from build123d import *

# Parameters (mm, degrees)
SKETCH1_W           = 95.25
SKETCH1_H           = 12.8
BOSS_EXTRUDE1_DEPTH = 161.88
SKETCH1_3_R         = 3.1
CUT_EXTRUDE1_DEPTH  = 20.2
SKETCH1_4_R         = 2.395
CUT_EXTRUDE2_DEPTH  = 21.5
CUT_EXTRUDE3_REACH  = 14.8
SKETCH2_R           = 9.525
CUT_EXTRUDE4_REACH  = 14.8
SKETCH3_R           = 3.265
SKETCH3_R_2         = 1.96
SKETCH3_R_3         = 2.56
SKETCH4_R           = 9.525
SKETCH4_R_2         = 5.09
CUT_EXTRUDE5_DEPTH  = 3.32
SKETCH5_R           = 5.31
CUT_EXTRUDE6_DEPTH  = 6.65
SKETCH6_R           = 1.965
CUT_EXTRUDE7_DEPTH  = 17.25
SKETCH7_R           = 1.97
CUT_EXTRUDE8_DEPTH  = 15.87
SKETCH9_R           = 9.5
CUT_EXTRUDE9_DEPTH  = 13.8000001


with BuildPart() as part:
    # Sketch1 → Boss-Extrude1 (new body)
    with BuildSketch(Plane.XY):
        with Locations((-282.25, -616.5)):
            Rectangle(SKETCH1_W, SKETCH1_H)
    extrude(amount=BOSS_EXTRUDE1_DEPTH)

    # Sketch1_3 → Cut-Extrude1 (cut)
    with BuildSketch(Plane.XY):
        with Locations((-307.5, -616.5)):
            Circle(SKETCH1_3_R)
        with Locations((-257, -616.5)):
            Circle(SKETCH1_3_R)
    extrude(amount=CUT_EXTRUDE1_DEPTH, mode=Mode.SUBTRACT)

    # Sketch1_4 → Cut-Extrude2 (cut)
    with BuildSketch(Plane.XY):
        with Locations((-244.2, -616.5)):
            Circle(SKETCH1_4_R)
        with Locations((-320.5, -616.5)):
            Circle(SKETCH1_4_R)
    extrude(amount=CUT_EXTRUDE2_DEPTH, mode=Mode.SUBTRACT)

    # Sketch2 → Cut-Extrude3 (cut, up to next)
    with BuildSketch(Plane(origin=(0, -610.1, 0), x_dir=(1, 0, 0), z_dir=(0, 1, 0)), mode=Mode.PRIVATE) as cut_extrude3_sk1:
        with Locations((-275.57, -124.135)):
            Circle(SKETCH2_R)
    cut_extrude3_tool1 = extrude(cut_extrude3_sk1.sketch, amount=-CUT_EXTRUDE3_REACH, mode=Mode.PRIVATE) & part.part
    add(cut_extrude3_tool1.solids().sort_by_distance((-275.57, -610.1, 124.135))[0], mode=Mode.SUBTRACT)
    # Sketch2 → Cut-Extrude3 (cut, up to next)
    with BuildSketch(Plane(origin=(0, -610.1, 0), x_dir=(1, 0, 0), z_dir=(0, 1, 0)), mode=Mode.PRIVATE) as cut_extrude3_sk2:
        with Locations((-275.57, -86.105)):
            Circle(SKETCH2_R)
    cut_extrude3_tool2 = extrude(cut_extrude3_sk2.sketch, amount=-CUT_EXTRUDE3_REACH, mode=Mode.PRIVATE) & part.part
    add(cut_extrude3_tool2.solids().sort_by_distance((-275.57, -610.1, 86.105))[0], mode=Mode.SUBTRACT)
    # Sketch2 → Cut-Extrude3 (cut, up to next)
    with BuildSketch(Plane(origin=(0, -610.1, 0), x_dir=(1, 0, 0), z_dir=(0, 1, 0)), mode=Mode.PRIVATE) as cut_extrude3_sk3:
        with BuildLine():
            Line((-269.505, 0), (-298.155, 0))
            Line((-298.155, 0), (-298.155, -25.4))
            ThreePointArc((-298.155, -25.4), (-297.276320344, -27.521320344), (-295.155, -28.4))
            Line((-295.155, -28.4), (-272.505, -28.4))
            ThreePointArc((-272.505, -28.4), (-270.383679656, -27.521320344), (-269.505, -25.4))
            Line((-269.505, -25.4), (-269.505, 0))
        make_face()
    cut_extrude3_tool3 = extrude(cut_extrude3_sk3.sketch, amount=-CUT_EXTRUDE3_REACH, mode=Mode.PRIVATE) & part.part
    add(cut_extrude3_tool3.solids().sort_by_distance((-283.83, -610.1, 14.135461))[0], mode=Mode.SUBTRACT)

    # Sketch3 → Cut-Extrude4 (cut, up to next)
    with BuildSketch(Plane(origin=(0, -610.1, 0), x_dir=(-1, 0, 0), z_dir=(0, 1, 0)), mode=Mode.PRIVATE) as cut_extrude4_sk1:
        with Locations((240.925, 140.49)):
            Circle(SKETCH3_R)
    cut_extrude4_tool1 = extrude(cut_extrude4_sk1.sketch, amount=-CUT_EXTRUDE4_REACH, mode=Mode.PRIVATE) & part.part
    add(cut_extrude4_tool1.solids().sort_by_distance((-240.925, -610.1, 140.49))[0], mode=Mode.SUBTRACT)
    # Sketch3 → Cut-Extrude4 (cut, up to next)
    with BuildSketch(Plane(origin=(0, -610.1, 0), x_dir=(-1, 0, 0), z_dir=(0, 1, 0)), mode=Mode.PRIVATE) as cut_extrude4_sk2:
        with Locations((253.55, 28.505)):
            Circle(SKETCH3_R)
    cut_extrude4_tool2 = extrude(cut_extrude4_sk2.sketch, amount=-CUT_EXTRUDE4_REACH, mode=Mode.PRIVATE) & part.part
    add(cut_extrude4_tool2.solids().sort_by_distance((-253.55, -610.1, 28.505))[0], mode=Mode.SUBTRACT)
    # Sketch3 → Cut-Extrude4 (cut, up to next)
    with BuildSketch(Plane(origin=(0, -610.1, 0), x_dir=(-1, 0, 0), z_dir=(0, 1, 0)), mode=Mode.PRIVATE) as cut_extrude4_sk3:
        with Locations((317.175, 111.08)):
            Circle(SKETCH3_R_2)
    cut_extrude4_tool3 = extrude(cut_extrude4_sk3.sketch, amount=-CUT_EXTRUDE4_REACH, mode=Mode.PRIVATE) & part.part
    add(cut_extrude4_tool3.solids().sort_by_distance((-317.175, -610.1, 111.08))[0], mode=Mode.SUBTRACT)
    # Sketch3 → Cut-Extrude4 (cut, up to next)
    with BuildSketch(Plane(origin=(0, -610.1, 0), x_dir=(-1, 0, 0), z_dir=(0, 1, 0)), mode=Mode.PRIVATE) as cut_extrude4_sk4:
        with Locations((321.975, 86.28)):
            Circle(SKETCH3_R_3)
    cut_extrude4_tool4 = extrude(cut_extrude4_sk4.sketch, amount=-CUT_EXTRUDE4_REACH, mode=Mode.PRIVATE) & part.part
    add(cut_extrude4_tool4.solids().sort_by_distance((-321.975, -610.1, 86.28))[0], mode=Mode.SUBTRACT)

    # Sketch4 → Cut-Extrude5 (cut)
    with BuildSketch(Plane(origin=(0, -610.1, 0), x_dir=(-1, 0, 0), z_dir=(0, 1, 0))):
        with Locations((253.55, 28.505)):
            Circle(SKETCH4_R)
        with Locations((240.925, 140.49)):
            Circle(SKETCH4_R_2)
    extrude(amount=-CUT_EXTRUDE5_DEPTH, mode=Mode.SUBTRACT)

    # Sketch5 → Cut-Extrude6 (cut)
    with BuildSketch(Plane.XZ.offset(622.9)):
        with Locations((-240.925, 140.49)):
            Circle(SKETCH5_R)
        with Locations((-253.55, 28.505)):
            Circle(SKETCH5_R)
    extrude(amount=-CUT_EXTRUDE6_DEPTH, mode=Mode.SUBTRACT)

    # Sketch6 → Cut-Extrude7 (cut)
    with BuildSketch(Plane.XY.offset(161.88)):
        with Locations((-310.715, -616.48)):
            Circle(SKETCH6_R)
        with Locations((-256.825, -616.48)):
            Circle(SKETCH6_R)
    extrude(amount=-CUT_EXTRUDE7_DEPTH, mode=Mode.SUBTRACT)

    # Sketch7 → Cut-Extrude8 (cut)
    with BuildSketch(Plane.ZY.offset(329.875)):
        with Locations((142.28, -616.5)):
            Circle(SKETCH7_R)
    extrude(amount=-CUT_EXTRUDE8_DEPTH, mode=Mode.SUBTRACT)

    # Sketch9 → Cut-Extrude9 (cut, through all)
    with BuildSketch(Plane.XZ.offset(622.9)):
        with Locations((-290.57, 38.77)):
            Circle(SKETCH9_R)
    extrude(amount=-CUT_EXTRUDE9_DEPTH, mode=Mode.SUBTRACT)


solid = part.part
The model under review builds one solid part; all positions refer to its coordinate system, in mm. A direction names the side the tool comes from. Coordinates: 2 decimals unless noted, no trailing zeros. Loops run counter-clockwise (first coordinate to the right, second up) from the corner with the lowest first, then second, coordinate; pieces in that order, holes last. Notation, with made-up numbers: M 79,-21 L 100,-21 A14 ccw 100,-14 Z; hole C 12,53.25 d7. An arc over 180 degrees is marked long. Put each result on its own line as item: value. Start each with the question number.
Q1. For faces 4 (the flat face through (-298.155, -616, 13)), 5 (the cylindrical face through (-321.019, -618.838, 10.599)), 6 (the cylindrical face through (-258.27, -615.15, 153.38)), list the 3-axis set-ups (+Z, -Z, +X, -X, +Y, -Y) from which the entire face can be reached by the end or side of a thin tool; tool diameter is ignored.
Q2. Wall thickness on line 1 (X direction, y = -616.5, z = 14.5) (3 decimals); line 2 (Y direction, x = -320.5, z = 17) (3 decimals); line 3 (Z direction, x = -241, y = -619.5): over which ranges is each line inside the solid? List them lowest first.
Q3. The part is to be moulded in two halves that separate along Y. For faces 1 (the cylindrical face through (-320.09, -616.41, 88.01)), 2 (the flat face through (-311, -616, 144.63)), 3 (the flat face through (-282.92, -610.1, 79.81)), say which applies: +Y half, -Y half, draft (parallel to the pull), parting line (faces both ways), or undercut.
Q4. Add section A-A (z = 111.08). Write out the cut boundary in (x, y) (3 decimals), and give its area (3 significant figures).
Q5. Clearance check with flat-ended pins moving along their axes: pin 1 (4 mm diameter, centred on x = -321.975, z = 86.28, fed in from -Y); pin 2 (4.5 mm diameter, centred on x = -244.2, y = -616.5, fed in from -Z); pin 3 (1.2 mm diameter, centred on x = -310, y = -617.5, fed in from +Z); pin 4 (4.5 mm diameter, centred on x = -256.825, y = -616.48, fed in from -Z). State where each tip first meets the part, or that it passes through.
Q6. Add section B-B (x = -287). Write out the cut boundary in (y, z).
Q7. Add section C-C (z = 35.5). Write out the cut boundary in (x, y) (3 decimals), and give its area (3 significant figures).
Answers:
1. face 4: -Z, +Y, -Y
1. face 5: -Z
1. face 6: +Z
2. line 1: x = -329.875 to -322.895, -318.105 to -310.6, -304.4 to -298.155, -269.505 to -260.1, -253.9 to -246.595, -241.805 to -234.625
2. line 2: y = -622.9 to -618.895, -614.105 to -610.1
2. line 3: z = 0 to 135.18, 145.8 to 161.88
3. face 1: draft
3. face 2: undercut
3. face 3: +Y half
4. outline: M -329.875,-622.9 L -319.135,-622.9 L -319.135,-610.1 L -329.875,-610.1 Z; M -315.215,-622.9 L -234.625,-622.9 L -234.625,-610.1 L -315.215,-610.1 Z
4. area: 1,170 mm^2
5. pin 1: passes through
5. pin 2: stops at z = 21.5
5. pin 3: stops at z = 144.63
5. pin 4: stops at z = 20.2
6. outline: M -622.9,28.4 L -610.1,28.4 L -610.1,29.97 L -622.9,29.97 Z; M -622.9,47.57 L -610.1,47.57 L -610.1,161.88 L -622.9,161.88 Z
7. outline: M -329.875,-622.9 L -299.489,-622.9 L -299.489,-610.1 L -329.875,-610.1 Z; M -281.651,-622.9 L -234.625,-622.9 L -234.625,-610.1 L -247.085,-610.1 L -247.085,-613.42 L -260.015,-613.42 L -260.015,-610.1 L -281.651,-610.1 Z
7. area: 948 mm^2
